Design review of the part built by this model. Coordinates are the model's own, in mm. Face numbers are marked on the shaded views. A direction names the side the tool comes from. Coordinates: 2 decimals unless noted, no trailing zeros. Order: outer loops, then holes, each group sorted by start corner. A loop starts at its lowest first (then second) coordinate and runs counter-clockwise, first axis right, second up. Notation, with made-up numbers: M 33,13 L 44,13 A18 cw 44,45 Z; hole C 88,-27 d9. An arc over 180 degrees is marked long. Answer as a JSON object with one key per item and string values.
from build123d import *

# Parameters (mm, degrees)
F0_R     = 3
F0_R_2   = 2.499
F1_DEPTH = 3.925
F2_R     = 3
F3_R     = 5
F4_R     = 3
F5_DEPTH = 1
F6_R     = 3
F6_R_2   = 2.499
F7_DEPTH = 1


# Not quite as in the source:
# - ends of sketch curves that miss each other by under 0.0002 mm in the source are joined


with BuildPart() as f1:
    # F0 (on Front) → F1 (new body, symmetric)
    with BuildSketch(Plane.XZ):
        Polygon((18.9613047033, 18.3160076926), (17.5273123959, 19.75), (-35.65, 19.75), (-35.65, 12.25), (14.4, 12.25), (28.1, -1.5000000006), (28.15, -19.7499999994), (28.15, -28.3999999994), (28.1, -46.65), (14.4, -60.4), (-35.65, -60.4), (-35.65, -67.9), (17.5273123959, -67.9), (18.9613047033, -66.4660076926), (35.65, -49.7773123959), (35.65, -28.4), (35.65, -19.75), (35.65, 1.6273123959), align=None)
        with Locations((-32.6, -64.15)):
            Circle(F0_R, mode=Mode.SUBTRACT)
        with Locations((-24.55, -64.15)):
            Circle(F0_R, mode=Mode.SUBTRACT)
        with Locations((-16.5, -64.15)):
            Circle(F0_R, mode=Mode.SUBTRACT)
        with Locations((-8.45, -64.15)):
            Circle(F0_R, mode=Mode.SUBTRACT)
        with Locations((-0.4, -64.15)):
            Circle(F0_R, mode=Mode.SUBTRACT)
        with Locations((7.65, -64.15)):
            Circle(F0_R, mode=Mode.SUBTRACT)
        with Locations((15.7, -64.15)):
            Circle(F0_R, mode=Mode.SUBTRACT)
        with BuildLine():
            ThreePointArc((19.6811007558, -64.5383771008), (18.6244738475, -61.4209978536), (15.5875186741, -60.1515818189))
            Line((15.5875186741, -60.1515818189), (22.1713217449, -53.5437502697))
            Line((22.1713217449, -53.5437502697), (22.9770950322, -52.735036204))
            Line((22.9770950322, -52.735036204), (28.7653917701, -46.9256142955))
            Line((28.7653917701, -46.9256142955), (34.7959320067, -49.4235458499))
            Line((34.7959320067, -49.4235458499), (27.2385163812, -56.9809614754))
            Line((27.2385163812, -56.9809614754), (26.4235246659, -57.7959531907))
            Line((26.4235246659, -57.7959531907), (19.6811007558, -64.5383771008))
        make_face(mode=Mode.SUBTRACT)
        Polygon((34.7959320067, -41.2253109008), (34.7959320067, -44.9256142955), (28.7681314859, -37.525), (28.7681314859, -33.8246890992), align=None, mode=Mode.SUBTRACT)
        Polygon((34.7959320067, -37.525), (28.7681314859, -30.7990158793), (28.7681314859, -27.436514941), (34.7959320067, -34.1624990617), align=None, mode=Mode.SUBTRACT)
        with Locations((-32.6, 16)):
            Circle(F0_R, mode=Mode.SUBTRACT)
        with Locations((-24.55, 16)):
            Circle(F0_R, mode=Mode.SUBTRACT)
        with Locations((-16.5, 16)):
            Circle(F0_R, mode=Mode.SUBTRACT)
        with Locations((-8.45, 16)):
            Circle(F0_R, mode=Mode.SUBTRACT)
        with Locations((-0.4, 16)):
            Circle(F0_R, mode=Mode.SUBTRACT)
        Polygon((28.7681314859, -20.7134831825), (28.7690151327, -17.3499982396), (34.7959320067, -10.625), (34.7959320067, -13.9874990617), (28.7685732445, -20.7129902561), align=None, mode=Mode.SUBTRACT)
        Polygon((28.7681314859, -10.625), (28.7698990648, -10.6228298581), (34.7959320067, -3.2243781985), (34.7959320067, -6.9246890992), (28.7694127753, -14.3237377999), (28.7698987796, -10.625), align=None, mode=Mode.SUBTRACT)
        with Locations((7.65, 16)):
            Circle(F0_R, mode=Mode.SUBTRACT)
        with Locations((15.7, 16)):
            Circle(F0_R, mode=Mode.SUBTRACT)
        with BuildLine():
            Line((22.176455222, 5.388598057), (15.5875186741, 12.0015818188))
            ThreePointArc((15.5875186741, 12.0015818188), (18.6244738475, 13.2709978536), (19.6811007558, 16.3883771008))
            Line((19.6811007558, 16.3883771008), (26.4364128886, 9.6330649683))
            Line((26.4364128886, 9.6330649683), (27.2385163814, 8.8309614755))
            Line((27.2385163814, 8.8309614755), (34.795932007, 1.2735458502))
            Line((34.795932007, 1.2735458502), (28.7653917699, -1.2243857048))
            Line((28.7653917699, -1.2243857048), (22.977095032, 4.5850362039))
            Line((22.977095032, 4.5850362039), (22.176455222, 5.388598057))
        make_face(mode=Mode.SUBTRACT)
        with Locations((-32.6, 16)):
            Circle(F0_R)
        with Locations((-32.6, 16)):
            Circle(F0_R_2, mode=Mode.SUBTRACT)
        with Locations((-24.55, 16)):
            Circle(F0_R)
        with Locations((-24.55, 16)):
            Circle(F0_R_2, mode=Mode.SUBTRACT)
        with Locations((-16.5, 16)):
            Circle(F0_R)
        with Locations((-16.5, 16)):
            Circle(F0_R_2, mode=Mode.SUBTRACT)
        with Locations((-0.4, 16)):
            Circle(F0_R)
        with Locations((-0.4, 16)):
            Circle(F0_R_2, mode=Mode.SUBTRACT)
        with Locations((7.65, 16)):
            Circle(F0_R)
        with Locations((7.65, 16)):
            Circle(F0_R_2, mode=Mode.SUBTRACT)
        with Locations((-8.45, 16)):
            Circle(F0_R)
        with Locations((-8.45, 16)):
            Circle(F0_R_2, mode=Mode.SUBTRACT)
        with Locations((15.7, 16)):
            Circle(F0_R)
        with Locations((15.7, 16)):
            Circle(F0_R_2, mode=Mode.SUBTRACT)
        with Locations((7.65, -64.15)):
            Circle(F0_R)
        with Locations((7.65, -64.15)):
            Circle(F0_R_2, mode=Mode.SUBTRACT)
        with Locations((15.7, -64.15)):
            Circle(F0_R)
        with Locations((15.7, -64.15)):
            Circle(F0_R_2, mode=Mode.SUBTRACT)
        with Locations((-0.4, -64.15)):
            Circle(F0_R)
        with Locations((-0.4, -64.15)):
            Circle(F0_R_2, mode=Mode.SUBTRACT)
        with Locations((-8.45, -64.15)):
            Circle(F0_R)
        with Locations((-8.45, -64.15)):
            Circle(F0_R_2, mode=Mode.SUBTRACT)
        with Locations((-16.5, -64.15)):
            Circle(F0_R)
        with Locations((-16.5, -64.15)):
            Circle(F0_R_2, mode=Mode.SUBTRACT)
        with Locations((-24.55, -64.15)):
            Circle(F0_R)
        with Locations((-24.55, -64.15)):
            Circle(F0_R_2, mode=Mode.SUBTRACT)
        with Locations((-32.6, -64.15)):
            Circle(F0_R)
        with Locations((-32.6, -64.15)):
            Circle(F0_R_2, mode=Mode.SUBTRACT)
        Polygon((22.9770950322, -52.735036204), (22.1713217449, -53.5437502697), (26.4235246659, -57.7959531907), (27.2385163812, -56.9809614754), align=None)
        Polygon((26.4364128886, 9.6330649683), (22.176455222, 5.388598057), (22.977095032, 4.5850362039), (27.2385163814, 8.8309614755), align=None)
    extrude(amount=F1_DEPTH, both=True)

    # F2
    f2_edges = [f1.edges().sort_by_distance(p)[0] for p in [
        (-35.65, 0, 19.75),
        (-35.65, 0, 12.25),
        (-35.65, 0, -60.4),
        (-35.65, 0, -67.9),
    ]]
    fillet(f2_edges, radius=F2_R)

    # F3
    f3_edges = [f1.edges().sort_by_distance(p)[0] for p in [
        (35.65, 0, 1.627312),
        (17.527312, 0, 19.75),
        (35.65, 0, -49.777312),
        (17.527312, 0, -67.9),
    ]]
    fillet(f3_edges, radius=F3_R)

    # F4 (on face) → F5 (cut)
    with BuildSketch(Plane.XZ.offset(3.925)):
        with Locations((-24.55, 16)):
            Circle(F4_R)
        with Locations((-16.5, 16)):
            Circle(F4_R)
        with Locations((-8.45, 16)):
            Circle(F4_R)
        with Locations((-0.4, 16)):
            Circle(F4_R)
        with Locations((7.65, 16)):
            Circle(F4_R)
        with Locations((15.7, 16)):
            Circle(F4_R)
        with Locations((-32.6, 16)):
            Circle(F4_R)
        with Locations((-32.6, -64.15)):
            Circle(F4_R)
        with Locations((-24.55, -64.15)):
            Circle(F4_R)
        with Locations((-16.5, -64.15)):
            Circle(F4_R)
        with Locations((-8.45, -64.15)):
            Circle(F4_R)
        with Locations((-0.4, -64.15)):
            Circle(F4_R)
        with Locations((7.65, -64.15)):
            Circle(F4_R)
        with Locations((15.7, -64.15)):
            Circle(F4_R)
    extrude(amount=-F5_DEPTH, mode=Mode.SUBTRACT)

    # F6 (on face) → F7 (cut)
    with BuildSketch(Plane(origin=(0, 3.925, 0), x_dir=(-1, 0, 0), z_dir=(0, 1, 0))):
        with Locations((-15.7, 16)):
            Circle(F6_R)
        with Locations((-15.7, 16)):
            Circle(F6_R_2, mode=Mode.SUBTRACT)
        with Locations((-7.65, 16)):
            Circle(F6_R)
        with Locations((-7.65, 16)):
            Circle(F6_R_2, mode=Mode.SUBTRACT)
        with Locations((0.4, 16)):
            Circle(F6_R)
        with Locations((0.4, 16)):
            Circle(F6_R_2, mode=Mode.SUBTRACT)
        with Locations((8.45, 16)):
            Circle(F6_R)
        with Locations((8.45, 16)):
            Circle(F6_R_2, mode=Mode.SUBTRACT)
        with Locations((16.5, 16)):
            Circle(F6_R)
        with Locations((16.5, 16)):
            Circle(F6_R_2, mode=Mode.SUBTRACT)
        with Locations((24.55, 16)):
            Circle(F6_R)
        with Locations((24.55, 16)):
            Circle(F6_R_2, mode=Mode.SUBTRACT)
        with Locations((32.6, 16)):
            Circle(F6_R)
        with Locations((32.6, 16)):
            Circle(F6_R_2, mode=Mode.SUBTRACT)
        with Locations((-15.7, -64.15)):
            Circle(F6_R)
        with Locations((-15.7, -64.15)):
            Circle(F6_R_2, mode=Mode.SUBTRACT)
        with Locations((-7.65, -64.15)):
            Circle(F6_R)
        with Locations((-7.65, -64.15)):
            Circle(F6_R_2, mode=Mode.SUBTRACT)
        with Locations((0.4, -64.15)):
            Circle(F6_R)
        with Locations((0.4, -64.15)):
            Circle(F6_R_2, mode=Mode.SUBTRACT)
        with Locations((8.45, -64.15)):
            Circle(F6_R)
        with Locations((8.45, -64.15)):
            Circle(F6_R_2, mode=Mode.SUBTRACT)
        with Locations((16.5, -64.15)):
            Circle(F6_R)
        with Locations((16.5, -64.15)):
            Circle(F6_R_2, mode=Mode.SUBTRACT)
        with Locations((24.55, -64.15)):
            Circle(F6_R)
        with Locations((24.55, -64.15)):
            Circle(F6_R_2, mode=Mode.SUBTRACT)
        with Locations((32.6, -64.15)):
            Circle(F6_R)
        with Locations((32.6, -64.15)):
            Circle(F6_R_2, mode=Mode.SUBTRACT)
    extrude(amount=-F7_DEPTH, mode=Mode.SUBTRACT)


solid = f1.part
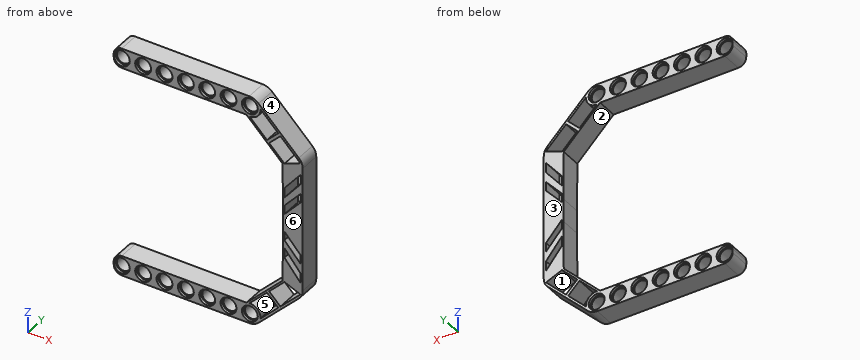
1) Add section D-D (x = 31.5). State the section outline as (y, z) points (3 decimals).
Taken from the geometry:
{"outline": "M -3.925,-53.927 L 3.925,-53.927 L 3.925,-52.719 L -3.925,-52.719 Z; M -3.925,-48.058 L 3.925,-48.058 L 3.925,-40.879 L -3.925,-40.879 Z; M -3.925,-37.179 L 3.925,-37.179 L 3.925,-33.847 L -3.925,-33.847 Z; M -3.925,-30.485 L 3.925,-30.485 L 3.925,-17.665 L -3.925,-17.665 Z; M -3.925,-14.303 L 3.925,-14.303 L 3.925,-10.971 L -3.925,-10.971 Z; M -3.925,-7.271 L 3.925,-7.271 L 3.925,-0.092 L -3.925,-0.092 Z; M -3.925,4.569 L 3.925,4.569 L 3.925,5.777 L -3.925,5.777 Z"}
2) Tool access review of the marked faces 1, 2 and 3: name each direction out of +Z, -Z, +X, -X, +Y, -Y from which nothing blocks a thin tool from reaching the whole face with its end or side.
Taken from the geometry:
{"face 1": "+Y, -Y", "face 2": "-X, +Y, -Y", "face 3": "+Z, -Z, +X, -X, +Y"}
3) To check wall thickness, follow L1, parallel to Z at x = 7.65, y = -3.6; L2, parallel to Z at x = -24.55, y = -1.4; L3, parallel to Z at x = -20, y = 0.25. State the ranges of each line that lie inside material, in increasing order.
Taken from the geometry:
{"L1": "z = -67.9 to -67.15, -61.15 to -60.4, 12.25 to 13, 19 to 19.75", "L2": "z = -67.9 to -66.65, -61.65 to -60.4, 12.25 to 13.5, 18.5 to 19.75", "L3": "z = -67.9 to -60.4, 12.25 to 19.75"}
4) Add section B-B (z = -29.5). State the section outline as (x, y) points (3 decimals), and give its area (3 significant figures).
Taken from the geometry:
{"outline": "M 28.147,-3.925 L 28.768,-3.925 L 28.768,3.925 L 28.147,3.925 Z; M 30.617,-3.925 L 35.65,-3.925 L 35.65,3.925 L 30.617,3.925 Z", "area": "44.4 mm2"}
5) Mouldability with a two-part tool opening along Z and no side actions: class the marked faces 4, 5 and 6 as released by +Z, released by -Z, zero draft, split by the parting line, or undercut.
Taken from the geometry:
{"face 4": "released by +Z", "face 5": "undercut", "face 6": "zero draft"}
6) Add section A-A (x = 7.65). Count the separate pieces of the cut face and the enclosed holes in it, and give its area (3 significant figures).
Taken from the geometry:
{"separate pieces": "4", "enclosed holes": "0", "area": "35.3 mm2"}
7) Insertion check: pin 1 Ø3 at (x, z) = (-25, 15) entering from -Y (3 decimals); pin 2 Ø4 at (y, z) = (0, 8) entering from -X; pin 3 Ø1.8 at (x, z) = (15.5, -63) entering from +Y; pin 4 Ø1.5 at (y, z) = (0, 10) entering from -X. Each pin has a flat end and moves straight along its axis. Give the tip position at first contact, or say it passes through.
Taken from the geometry:
{"pin 1": "stops at y = -2.925", "pin 2": "stops at x = 16.64", "pin 3": "passes through", "pin 4": "stops at x = 15.89"}
